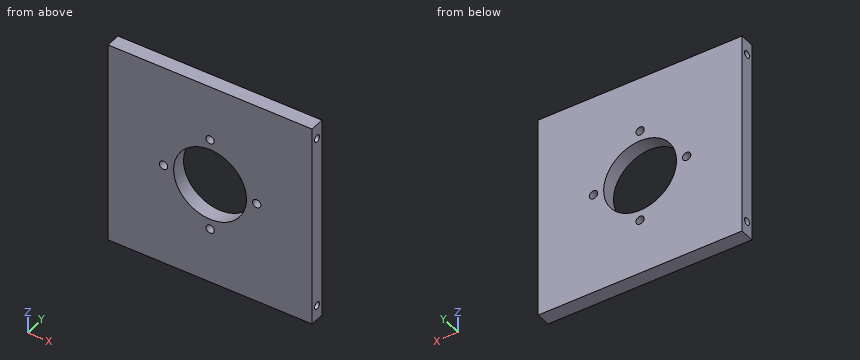
Autodesk Inventor part; units mm, degrees
ref_plane "Work Plane2" through (0, 0, -35) normal (-1, 0, 0) x (0, 0, 1)
ref_plane "YZ Plane" through (0, 0, 0) normal (1, 0, 0) x (0, 1, 0)
ref_plane "XZ Plane" through (0, 0, 0) normal (0, 1, 0) x (-1, 0, 0)
sketch "Sketch1" plane through (0, 0, 0) normal (0, 1, 0) x (-1, 0, 0)
  line L0 (35, 35) -> (-35, 35)
  line L1 (-35, 35) -> (-35, -35)
  line L2 (-35, -35) -> (35, -35)
  line L3 (35, -35) -> (35, 35)
  line L4 (0, -49) -> (0, 49)
  line L5 (49, 0) -> (-49, 0)
  point P0 (0, 0)
  dimension "d0" = 70
  dimension "d1" = 70
  dimension "d2" = 70
extrude "Extrusion1" add sketch "Sketch1" along normal blind 5
sketch "Sketch2" plane through (35, 0, 35) normal (1, 0, 0) x (0, 0, -1)
  line L0 (0, 0) -> (70, 0)
  line L1 (70, 0) -> (70, 5)
  line L2 (35, 0) -> (35, 5)
  line L3 (0, 5) -> (70, 5)
  point P0 (65, 2.5)
  point P1 (5, 2.5)
  dimension "d5" = 2.5
  dimension "d6" = 5
hole "Hole1" at (35, 2.5, -30) at (35, 2.5, 30) direction (-1, 0, 0) diameter 2.459 depth 8.8 tip angle 118
sketch "Sketch3" plane through (0, 5, 0) normal (0, 1, 0) x (1, 0, 0)
  point P0 (0, 0)
  point P1 (0, 0)
hole "Hole2" at (0, 5, 0) direction (0, -1, 0) diameter 25 depth 10 tip angle 118
sketch "Sketch4" plane through (0, 5, 0) normal (0, 1, 0) x (1, 0, 0)
  point P0 (0, 0)
  point P1 (16, 0)
  point P2 (0, 16)
  point P3 (-16, 0)
  point P4 (0, -16)
  dimension "d21" = 16
  dimension "d24" = 360
sketch "Sketch5" plane through (0, 5, 0) normal (0, 1, 0) x (1, 0, 0)
  point P0 (0, 0)
hole "Hole3" at (-16, 5, 0) at (0, 5, -16) at (0, 5, 16) at (16, 5, 0) direction (0, -1, 0) diameter 2.85 depth 10.4 tip angle 118
ref_plane "Work Plane2" through (0, 0, -35) normal (-1, 0, 0) x (0, 0, 1)
mirror "Mirror2" about plane through (0, 0, -35) normal (-1, 0, 0) of "Hole1"
properties part number "상판" material "Aluminum 6061-AHC"
Could you check a few things on this model? Use its own coordinates, in mm. Give positions to 0.01 mm unless a question says otherwise; leave off trailing zeros. Write each loop counter-clockwise with the first axis right and the second up, starting at its lowest first coordinate (ties: lowest second). Pieces come first, ordered by that corner, then holes. Notation, with made-up numbers: (12.25, -1) -> (59.25, -1) arc R27 ccw to (59.25, 15) -> close; hole circle Ø6 at (58.5, 82). An arc over 180 degrees is marked (long way). Write each question's results on one line, items separated by ' | '.
1. Will these pins go through, and if not, where does the flat tip stop? pin 1 Ø2 at (y, z) = (2.5, 30) entering from -X; pin 2 Ø22.5 at (x, z) = (0, 0) entering from +Y.
Check sheet entries:
pin 1: stops at x = -26.06 | pin 2: passes through
2. I want a section at B-B, the plane z = -10. Write out the boundary of the cut face in (x, y), then the cut area to 3 significant figures.
Check sheet entries:
outline: (-35, 0) -> (-7.5, 0) -> (-7.5, 5) -> (-35, 5) -> close; (7.5, 0) -> (35, 0) -> (35, 5) -> (7.5, 5) -> close | area: 275 mm²
3. I want a section at C-C, the plane x = 16. Write out the boundary of the cut face in (y, z) (3 decimals).
Check sheet entries:
outline: (0, -35) -> (5, -35) -> (5, -1.425) -> (0, -1.425) -> close; (0, 1.425) -> (5, 1.425) -> (5, 35) -> (0, 35) -> close
4. I need wall thicknesses on L1, parallel to Z at x = 28.5, y = 2.5; L2, parallel to X at y = 3.4, z = 0 (3 decimals). Which ranges of each line are inside material? Lowest first, please.
Check sheet entries:
L1: z = -35 to -31.23, -28.77 to 28.77, 31.23 to 35 | L2: x = -35 to -17.425, -14.575 to -12.5, 12.5 to 14.575, 17.425 to 35
5. I want a section at A-A, the plane x = 0. Write out the boundary of the cut face in (y, z) (3 decimals), then the cut area to 4 significant figures.
Check sheet entries:
outline: (0, -35) -> (5, -35) -> (5, -17.425) -> (0, -17.425) -> close; (0, -14.575) -> (5, -14.575) -> (5, -12.5) -> (0, -12.5) -> close; (0, 12.5) -> (5, 12.5) -> (5, 14.575) -> (0, 14.575) -> close; (0, 17.425) -> (5, 17.425) -> (5, 35) -> (0, 35) -> close | area: 196.5 mm²
